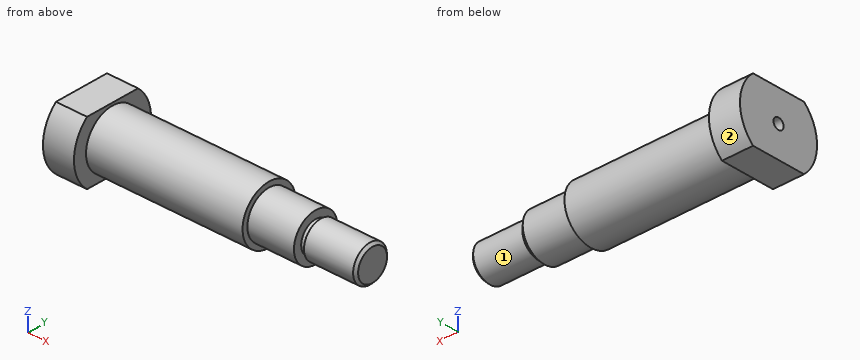
```python
from build123d import *

# Parameters (mm, degrees)
CHAMFER1_SIZE             = 1
CUT_EXTRUDE1_DEPTH        = 12
M5X0_8_TAPPED_HOLE1_D     = 4.2
M5X0_8_TAPPED_HOLE1_DEPTH = 63
M5X0_8_TAPPED_HOLE1_TIP   = 1.2618073


with BuildPart() as part:
    # Sketch1 → Revolve1 (revolve)
    with BuildSketch(Plane.XY, mode=Mode.PRIVATE) as revolve1_sk:
        Polygon((17, 11), (-43.5, 11), (-43.5, 16), (-55.5, 16), (-55.5, 0), (57, 0), (57, 7), (37, 7), (37, 6), (35, 6), (35, 9), (17, 9), align=None)
    revolve(revolve1_sk.sketch.rotate(Axis((57, 0, 0), (-1, 0, 0)), 90), axis=Axis((57, 0, 0), (-1, 0, 0)))

    # Chamfer1
    chamfer1_edges = [part.edges().sort_by_distance(p)[0] for p in [
        (57, 0, 7),
    ]]
    chamfer(chamfer1_edges, length=CHAMFER1_SIZE)

    # Sketch2 → Cut-Extrude1 (cut)
    with BuildSketch(Plane.ZY.offset(55.5)):
        with BuildLine():
            Line((12, 10.583005244), (12, -10.583005244))
            ThreePointArc((12, -10.583005244), (16, 0), (12, 10.583005244))
        make_face()
        with BuildLine():
            Line((-12, 10.583005244), (-12, -10.583005244))
            ThreePointArc((-12, -10.583005244), (-16, 0), (-12, 10.583005244))
        make_face()
    extrude(amount=-CUT_EXTRUDE1_DEPTH, mode=Mode.SUBTRACT)

    # M5x0.8 Tapped Hole1
    with Locations(Plane.ZY.offset(55.5)):
        with Locations((0, 0)):
            Hole(M5X0_8_TAPPED_HOLE1_D / 2, depth=M5X0_8_TAPPED_HOLE1_DEPTH)
            with Locations((0, 0, -(M5X0_8_TAPPED_HOLE1_DEPTH + M5X0_8_TAPPED_HOLE1_TIP / 2))):  # 118° drill point
                Cone(0, M5X0_8_TAPPED_HOLE1_D / 2, M5X0_8_TAPPED_HOLE1_TIP, mode=Mode.SUBTRACT)


solid = part.part
```
The listing builds one solid part. Answer for the finished solid, in the listing's coordinates (mm). Face numbers are marked on the shaded views. A direction names the side the tool comes from. Give positions to 0.01 mm unless a question says otherwise; leave off trailing zeros. Write each loop counter-clockwise with the first axis right and the second up, starting at its lowest first coordinate (ties: lowest second). Pieces come first, ordered by that corner, then holes. Notation, with made-up numbers: (41, -1) - (94, -1) arc R9 cw to (94, 14) - close; hole circle Ø6 at (22, 60). An arc over 180 degrees is marked (long way). Use one line per item in the form item = value. Start each with the question number.
1) Find section B-B on y = 8. Determine the outline of the cut face in (x, z), plus the area to 3 significant figures.
2) Flat-ended cylindrical pins translate along their axes: pin 1 Ø2 at (y, z) = (5, -5.5) entering from +X; pin 2 Ø2.5 at (y, z) = (0, 0) entering from -X; pin 3 Ø8 at (x, z) = (-20.5, 1.5) entering from -Y; pin 4 Ø3 at (y, z) = (2, 6.5) entering from +X. Find the tip coordinate at first contact, or state that the pin passes through.
3) Find section A-A on x = -0.5. Determine the outline of the cut face in (y, z), plus the area to 3 significant figures.
4) Find section D-D on y = 13. Determine the outline of the cut face in (x, z), plus the area to 3 significant figures.
5) Consider line 1 along Y through (x, z) = (-6, 0); line 2 along X through (y, z) = (-13, -7.5); line 3 along Z through (x, y) = (-35, -1). Determine where each line is inside the solid, lowest interval first. Write a range as from..to.
6) A tool of negligible diameter and unlimited length cuts with its end or side. For the marked faces 1 and 2, from which of +Z, -Z, +X, -X, +Y, -Y can it reach the whole face along a straight path? Write none if from no direction.
7) Find section C-C on x = 39. Determine the outline of the cut face in (y, z).
Geometry results:
q1.outline = (-55.5, -12) - (-43.5, -12) - (-43.5, -7.55) - (17, -7.55) - (17, -4.12) - (35, -4.12) - (35, 4.12) - (17, 4.12) - (17, 7.55) - (-43.5, 7.55) - (-43.5, 12) - (-55.5, 12) - close
q1.area = 1,350 mm2
q2.pin_1 = 56.57
q2.pin_2 = 8.01
q2.pin_3 = -11
q2.pin_4 = 57
q3.outline = circle Ø22 at (0, 0); hole circle Ø4.2 at (0, 0)
q3.area = 366 mm2
q4.outline = (-55.5, -9.33) - (-43.5, -9.33) - (-43.5, 9.33) - (-55.5, 9.33) - close
q4.area = 224 mm2
q5.line_1 = -11..-2.1, 2.1..11
q5.line_2 = -55.5..-43.5
q5.line_3 = -10.95..-1.85, 1.85..10.95
q6.face_1 = +X
q6.face_2 = +X, -X, +Y
q7.outline = circle Ø14 at (0, 0)
